Job drawing, mm, ordinate dimensions from the low corner. One solid piece. Coordinates: 2 decimals unless noted, no trailing zeros. Write each loop counter-clockwise with the first axis right and the second up, starting at its lowest first coordinate (ties: lowest second). Pieces come first, ordered by that corner, then holes. Notation, with made-up numbers: (59.25, -27) -> (100.25, -27) arc R18 cw to (100.25, -19) -> close; hole circle Ø11 at (10.5, 42.5). An arc over 180 degrees is marked (long way). One line per question, with ' | ' between items. Start each with the question number.
Item 1: Saw through at C-C (z = 15). List the corners of the cut face in (x, y), and give its area (3 significant figures).
Item 2: Saw through at A-A (x = 108.1). List the corners of the cut face in (y, z), and give its area (3 significant figures).
Item 3: Probe probe 1 along X at (y, z) = (3.75, 15); probe 2 along Z at (x, y) = (108.1, 2.25); probe 3 along Z at (x, y) = (60.5, 1.25) (3 decimals). List the from-to ranges inside material, lowest first. Write a range as [from, to].
Item 4: Saw through at B-B (y = 4.75). List the corners of the cut face in (x, z) (3 decimals), and give its area (3 significant figures).
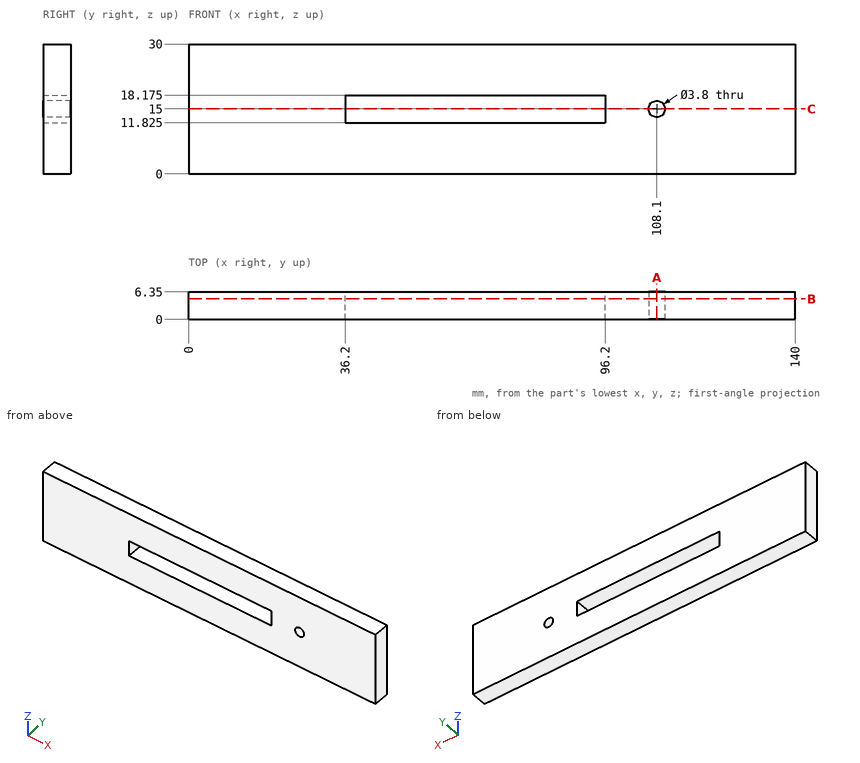
From the geometry:
1) outline: (0, 0) -> (36.2, 0) -> (36.2, 6.35) -> (0, 6.35) -> close; (96.2, 0) -> (106.2, 0) -> (106.2, 6.35) -> (96.2, 6.35) -> close; (110, 0) -> (140, 0) -> (140, 6.35) -> (110, 6.35) -> close | area: 484 mm2
2) outline: (0, 0) -> (6.35, 0) -> (6.35, 13.1) -> (0, 13.1) -> close; (0, 16.9) -> (6.35, 16.9) -> (6.35, 30) -> (0, 30) -> close | area: 166 mm2
3) probe 1: [0, 36.2], [96.2, 106.2], [110, 140] | probe 2: [0, 13.1], [16.9, 30] | probe 3: [0, 11.825], [18.175, 30]
4) outline: (0, 0) -> (140, 0) -> (140, 30) -> (0, 30) -> close; hole (36.2, 11.825) -> (96.2, 11.825) -> (96.2, 18.175) -> (36.2, 18.175) -> close; hole circle Ø3.8 at (108.1, 15) | area: 3,810 mm2
